The listing builds one solid part. Answer for the finished solid, in the listing's coordinates (mm). Face numbers are marked on the shaded views. A direction names the side the tool comes from. Coordinates: 2 decimals unless noted, no trailing zeros. Order: outer loops, then holes, each group sorted by start corner. A loop starts at its lowest first (then second) coordinate and runs counter-clockwise, first axis right, second up. Notation, with made-up numbers: (68, 17) -> (105, 17) arc R23 ccw to (105, 34) -> close; hole circle Ø10 at (74.5, 62.25). An arc over 180 degrees is marked (long way). Write item = value, one per line.
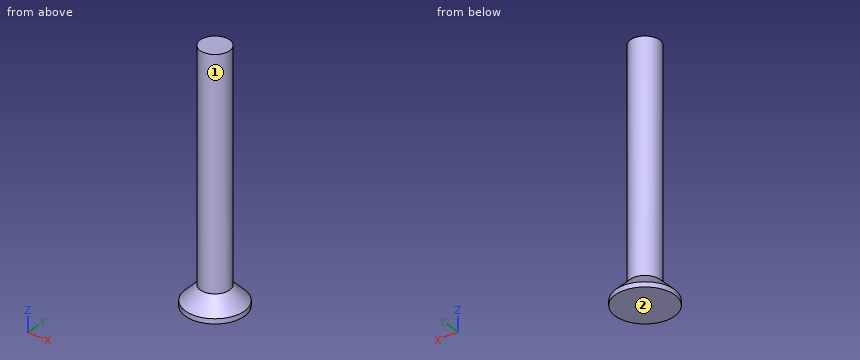
Autodesk Inventor part; units mm, degrees
ref_plane "YZ Plane" through (0, 0, 0) normal (1, 0, 0) x (0, 1, 0)
ref_plane "XZ Plane" through (0, 0, 0) normal (0, 1, 0) x (-1, 0, 0)
ref_plane "XY Plane" through (0, 0, 0) normal (0, 0, 1) x (1, 0, 0)
sketch "スケッチ1" plane through (0, 0, 0) normal (0, 0, 1) x (1, 0, 0)
  circle A0 centre (0, 0) radius 1.5
  dimension "d0" = 3
extrude "押し出し1" add sketch "スケッチ1" along normal blind 25
sketch "スケッチ2" plane through (0, 0, 0) normal (0, 0, -1) x (-1, 0, 0)
  circle A0 centre (0, 0) radius 3
  dimension "d3" = 6
extrude "押し出し2" add sketch "スケッチ2" against normal blind 2
thread "ねじ1"
chamfer "面取り1" distance 1.5 angle 45 1 edges at (3, 0, 2)
properties part number "ネジ皿m3,26" material "鋼、高強度、低合金"
Q1. Each of these flat-tipped pins is pushed along its axis until it touches: pin 1 Ø2 at (y, z) = (0.5, 5.5) entering from +X; pin 2 Ø1.5 at (x, z) = (1, 20.5) entering from +Y; pin 3 Ø1 at (x, z) = (-1, 9) entering from -Y. Where does it stop, or does it pass through?
The answers:
pin_1 = 1.5
pin_2 = 1.48
pin_3 = -1.41
Q2. A tool of negligible diameter and unlimited length cuts with its end or side. For the marked faces 1 and 2, from which of +Z, -Z, +X, -X, +Y, -Y can it reach the whole face along a straight path? Write none if from no direction.
The answers:
face_1 = +Z
face_2 = -Z, +X, -X, +Y, -Y
Q3. Section C-C, the plane z = 17 is taken. Give the vertices of the cut face in (x, y).
The answers:
outline = circle Ø3 at (0, 0)
Q4. Find the intervals of material crossed by line 1 along Z through (x, y) = (-1.2, 1.6); line 2 along Z through (x, y) = (-2.1, -1.55); line 3 along Y through (x, z) = (-0.4, 20.5), in increasing order.
The answers:
line_1 = 0 to 1.5
line_2 = 0 to 0.89
line_3 = -1.45 to 1.45
